from build123d import *

# Parameters (mm, degrees)
F0_W = 22.9998864233
F0_H = 10.1898247376


with BuildPart() as f1:
    # F0 (on Front) → F1 (revolve)
    with BuildSketch(Plane.XZ):
        Polygon((-40.3225906193, 0), (-37.2656472027, 0), (-37.2656472027, 10.1898247376), (-60.2655336261, 10.1898247376), (-60.2655336261, 0), align=None)
        Polygon((-37.2656472027, 0), (-18.0505476892, 0), (-18.0505476892, 20.3796494752), (-37.2656472027, 20.3796494752), (-37.2656472027, 10.1898247376), align=None)
        Polygon((-18.0505476892, 0), (0, 0), (0, 28.5315085202), (-18.0505476892, 28.5315085202), (-18.0505476892, 20.3796494752), align=None)
        Polygon((0, 28.5315085202), (0, 0), (18.0505476892, 0), (18.0505476892, 20.3796494752), (18.0505476892, 28.5315085202), align=None)
        Polygon((18.0505476892, 20.3796494752), (18.0505476892, 0), (37.2656472027, 0), (37.2656472027, 10.1898247376), (37.2656472027, 20.3796494752), align=None)
        with Locations((48.7655904144, 5.0949123688)):
            Rectangle(F0_W, F0_H)
    revolve(axis=Axis((3.493655473, 0, 0), (1, 0, 0)))


solid = f1.part
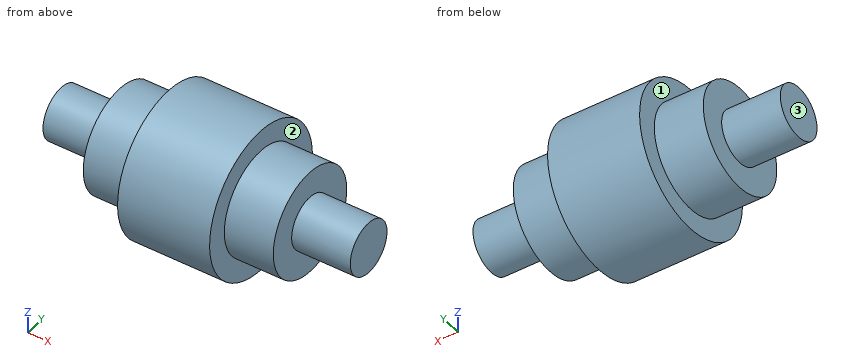
Check sheet for the modelled part. Datum: model origin and axes. Units: mm. Face numbers are marked on the shaded views. A direction names the side the tool comes from. Round coordinates to 2 decimals unless told otherwise and drop trailing zeros. Order: outer loops, then holes, each group sorted by start corner. A loop starts at its lowest first (then second) coordinate and runs counter-clockwise, first axis right, second up.
Q1. Depth check by flat-ended pin: P1, Ø3, axis at x = -6.5, y = -9, coming from the -Z side; P2, Ø8, axis at x = 9.5, z = 21, coming from the +Y side; P3, Ø4, axis at y = 22, z = 6.5, coming from the -X side. Enter the tip coordinate at first touch or a pass-through.
Filled sheet:
P1: stops at z = -27.53
P2: stops at y = 22.91
P3: stops at x = -18.05
Q2. Scan lines: L1, parallel to X at y = -19.5, z = 20.5; L2, parallel to X at y = -11.5, z = -2.5; L3, parallel to Y at x = -9, z = 9.5. Record each from-to range of solid material in increasing order.
Filled sheet:
L1: x = -18.05 to 18.05
L2: x = -37.27 to 37.27
L3: y = -26.9 to 26.9
Q3. Cross-section at A-A, the plane y = 0. Enter the section's corners in (x, z), plus the area to 3 significant figures.
Filled sheet:
outline: (-60.27, -10.19) - (-37.27, -10.19) - (-37.27, -20.38) - (-18.05, -20.38) - (-18.05, -28.53) - (18.05, -28.53) - (18.05, -20.38) - (37.27, -20.38) - (37.27, -10.19) - (60.27, -10.19) - (60.27, 10.19) - (37.27, 10.19) - (37.27, 20.38) - (18.05, 20.38) - (18.05, 28.53) - (-18.05, 28.53) - (-18.05, 20.38) - (-37.27, 20.38) - (-37.27, 10.19) - (-60.27, 10.19) - close
area: 4,560 mm2
Q4. Cross-section at C-C, the plane x = -31.5. Enter the section's corners in (y, z), plus the area to 3 significant figures.
Filled sheet:
outline: circle Ø40.76 at (0, 0)
area: 1,300 mm2
Q5. Set-up check for the marked faces 1, 2 and 3: record each of +Z, -Z, +X, -X, +Y, -Y from which the full face is reachable in a straight line by a thin tool's end or side.
Filled sheet:
face 1: -X
face 2: +X
face 3: +Z, -Z, -X, +Y, -Y
Q6. Cross-section at D-D, the plane x = 50. Enter the section's corners in (y, z).
Filled sheet:
outline: circle Ø20.38 at (0, 0)
